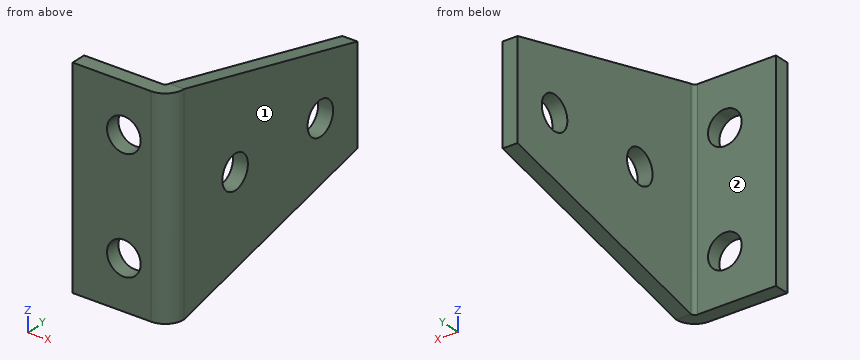
from build123d import *

# Parameters (mm, degrees)
EXTRUDE_THIN1_DEPTH     = 44.45
CUT_EXTRUDE2_DEPTH      = 120.051916196
CUT_EXTRUDE2_DEPTH_BACK = 120.051916196
SKETCH3_R               = 7.14375
CUT_EXTRUDE3_DEPTH      = 120.051916196
SKETCH4_R               = 7.14375
CUT_EXTRUDE4_DEPTH      = 116.615348246


with BuildPart() as part:
    # Sketch1 → Extrude-Thin1 (new, symmetric)
    with BuildSketch(Plane.XY):
        with BuildLine():
            Line((-41.275, 0), (-7.9375, 0))
            ThreePointArc((-7.9375, 0), (-2.324839924, 2.324839924), (0, 7.9375))
            Line((0, 7.9375), (0, 104.775))
            Line((0, 104.775), (-6.35, 104.775))
            Line((-6.35, 104.775), (-6.35, 7.9375))
            ThreePointArc((-6.35, 7.9375), (-6.814967985, 6.814967985), (-7.9375, 6.35))
            Line((-7.9375, 6.35), (-41.275, 6.35))
            Line((-41.275, 6.35), (-41.275, 0))
        make_face()
    extrude(amount=EXTRUDE_THIN1_DEPTH, both=True)

    # Sketch2 → Cut-Extrude2 (cut, two sides: drawn at the far end of the back side and taken through both)
    with BuildSketch(Plane.ZY.offset(6.35).offset(-CUT_EXTRUDE2_DEPTH_BACK)):
        Polygon((-109.618200913, -257.07985038), (-44.45, 7.9375), (-20.6375, 104.775), (20.6375, 104.775), (44.45, 7.9375), (109.618200913, -257.07985038), (109.618200913, 288.744628415), (-109.618200913, 288.744628415), align=None)
    extrude(amount=CUT_EXTRUDE2_DEPTH + CUT_EXTRUDE2_DEPTH_BACK, mode=Mode.SUBTRACT)

    # Sketch3 → Cut-Extrude3 (cut, through all)
    with BuildSketch(Plane.ZY.offset(6.35)):
        with Locations((0, 84.1375)):
            Circle(SKETCH3_R)
        with Locations((0, 36.5125)):
            Circle(SKETCH3_R)
    extrude(amount=-CUT_EXTRUDE3_DEPTH, mode=Mode.SUBTRACT)

    # Sketch4 → Cut-Extrude4 (cut, through all)
    with BuildSketch(Plane(origin=(0, 6.35, 0), x_dir=(1, 0, 0), z_dir=(0, 1, 0))):
        with Locations(Location((-19.52625, 23.8125, 0), (0, 0, 270))):
            Circle(SKETCH4_R)
        with Locations(Location((-19.52625, -23.8125, 0), (0, 0, 270))):
            Circle(SKETCH4_R)
    extrude(amount=-CUT_EXTRUDE4_DEPTH, mode=Mode.SUBTRACT)


solid = part.part
Input: part model. Units: mm. Frame: model coordinates. Face numbers are marked on the shaded views. A direction names the side the tool comes from. Round coordinates to 2 decimals unless told otherwise and drop trailing zeros. Write each loop counter-clockwise with the first axis right and the second up, starting at its lowest first coordinate (ties: lowest second). Pieces come first, ordered by that corner, then holes.
1) Cut plane A-A (z = 0). Count the separate pieces of the cut face and the enclosed holes in it, then the cut area to 3 significant figures.
2) Contact query for flat-ended pins moving along their axis: P1, Ø4, axis at x = -13, z = 25, coming from the +Y side; P2, Ø1, axis at x = -22, z = 29.5, coming from the -Y side; P3, Ø23, axis at y = 84.14, z = 0, coming from the -X side. Output: stop coordinate, or through.
3) Reachability of the marked faces 1 and 2 from +Z, -Z, +X, -X, +Y, -Y: full face, straight path, thin tool, end or side. Return the list, or none.
4) Cut plane B-B (y = 38). Return the cut outline in (x, z).
5) Cut plane C-C (x = -17.5). Return the cut outline in (y, z).
6) Ray query, L1, parallel to Y at x = -2, z = 0 (3 decimals); L2, parallel to X at y = 25.5, z = 32.5. Return the intervals inside material, ascending.
Geometry says:
1. separate pieces: 3
1. enclosed holes: 0
1. area: 693 mm2
2. P1: stops at y = 6.35
2. P2: passes through
2. P3: stops at x = -6.35
3. face 1: +Z, -Z, +X, +Y, -Y
3. face 2: +Z, -Z, -X, +Y
4. outline: (-6.35, -37.06) - (0, -37.06) - (0, -6.99) - (-6.35, -6.99) - close; (-6.35, 6.99) - (0, 6.99) - (0, 37.06) - (-6.35, 37.06) - close
5. outline: (0, -44.45) - (6.35, -44.45) - (6.35, -30.66) - (0, -30.66) - close; (0, -16.96) - (6.35, -16.96) - (6.35, 16.96) - (0, 16.96) - close; (0, 30.66) - (6.35, 30.66) - (6.35, 44.45) - (0, 44.45) - close
6. L1: y = 2.67 to 29.369, 43.656 to 76.994, 91.281 to 104.775
6. L2: x = -6.35 to 0
